from build123d import *

# Parameters (mm, degrees)
SKETCH1_R                = 2.54
BOSS_EXTRUDE1_DEPTH      = 5.08
BOSS_EXTRUDE1_DEPTH_BACK = 5.08
CUT_EXTRUDE1_DEPTH       = 8.981097998
CUT_EXTRUDE1_DEPTH_BACK  = 4.81


with BuildPart() as part:
    # Sketch1 → Boss-Extrude1 (new body, two sides)
    with BuildSketch(Plane(origin=(0, 0, 0), x_dir=(1, 0, 0), z_dir=(0, 1, 0))) as boss_extrude1_sk:
        with BuildLine():
            Line((-2.006502941, 3.238834041), (-11.917388437, -2.901097998))
            Line((-11.917388437, -2.901097998), (-16.997388437, -2.901097998))
            Line((-16.997388437, -2.901097998), (-16.997388437, -7.981097998))
            Line((-16.997388437, -7.981097998), (-11.917388437, -7.981097998))
            Line((-11.917388437, -7.981097998), (0, -3.81))
            Line((0, -3.81), (11.917388437, -7.981097998))
            Line((11.917388437, -7.981097998), (16.997388437, -7.981097998))
            Line((16.997388437, -7.981097998), (16.997388437, -2.901097998))
            Line((16.997388437, -2.901097998), (11.917388437, -2.901097998))
            Line((11.917388437, -2.901097998), (2.006502941, 3.238834041))
            ThreePointArc((2.006502941, 3.238834041), (0, 3.81), (-2.006502941, 3.238834041))
        make_face()
        Circle(SKETCH1_R, mode=Mode.SUBTRACT)
    extrude(amount=BOSS_EXTRUDE1_DEPTH)
    extrude(boss_extrude1_sk.sketch, amount=-BOSS_EXTRUDE1_DEPTH_BACK)

    # Sketch2 → Cut-Extrude1 (cut, two sides)
    with BuildSketch(Plane.XY) as cut_extrude1_sk:
        Polygon((-11.917388437, -6.525255909), (-11.917388437, -2.478330742), (-9.439057695, 0), (9.439057695, 0), (11.917388437, -2.478330742), (11.917388437, -6.525255909), align=None)
        Polygon((-18.093487835, 0), (-11.917388437, 0), (-7.769454267, 4.147934171), (7.769454267, 4.147934171), (11.917388437, 0), (18.118549734, 0), (18.118549734, 7.57171578), (-18.093487835, 7.57171578), align=None)
    extrude(amount=CUT_EXTRUDE1_DEPTH, mode=Mode.SUBTRACT)
    extrude(cut_extrude1_sk.sketch, amount=-CUT_EXTRUDE1_DEPTH_BACK, mode=Mode.SUBTRACT)

    # Sketch3 → Cut-Revolve1 (revolve, cut)
    with BuildSketch(Plane.XY.offset(5.441097998)):
        with BuildLine():
            Line((-12.967633979, -0.885782562), (-12.851197898, -0.885782562))
            Line((-12.851197898, -0.885782562), (-12.851197898, 1.801061794))
            Line((-12.851197898, 1.801061794), (-18.158310447, 1.801061794))
            Line((-18.158310447, 1.801061794), (-18.158310447, -2.54))
            Line((-18.158310447, -2.54), (-16.997388437, -2.54))
            ThreePointArc((-16.997388437, -2.54), (-15.537067777, -0.361964398), (-12.967633979, -0.885782562))
        make_face()
        with BuildLine():
            Line((12.851197898, -0.885782562), (12.851197898, 1.801061794))
            Line((12.851197898, 1.801061794), (18.158310447, 1.801061794))
            Line((18.158310447, 1.801061794), (18.158310447, -2.54))
            Line((18.158310447, -2.54), (16.997388437, -2.54))
            ThreePointArc((16.997388437, -2.54), (15.537067777, -0.361964398), (12.967633979, -0.885782562))
            Line((12.967633979, -0.885782562), (12.851197898, -0.885782562))
        make_face()
    revolve(axis=Axis((-16.997388437, -2.54, 5.441097998), (1, 0, 0)), mode=Mode.SUBTRACT)


solid = part.part
Verification items for the finished model (mm, model axes). A direction names the side the tool comes from. Coordinates: 2 decimals unless noted, no trailing zeros. Order: outer loops, then holes, each group sorted by start corner. A loop starts at its lowest first (then second) coordinate and runs counter-clockwise, first axis right, second up. Notation, with made-up numbers: M 14.25,-27 L 24.25,-27 A5 cw 24.25,-23 Z; hole C -9.5,69 d10. An arc over 180 degrees is marked long. One line per item, written item: value. Start each with the question number.
Item 1: Sectioned sample at D-D on x = -13.5. Record the cut outline in (y, z).
Item 2: Depth check by flat-ended pin: P1, Ø6, axis at x = -3, z = 2.5, coming from the -Y side; P2, Ø3, axis at y = 0.5, z = 6.5, coming from the +X side; P3, Ø0.5, axis at x = -12.5, z = 5.5, coming from the +Y side. Enter the tip coordinate at first touch or a pass-through.
Item 3: Sectioned sample at C-C on z = 2. Record the cut outline in (x, y).
Item 4: Access from +Z, -Z, +X, -X, +Y, -Y to the whole of each face (thin tool, end or side, straight path). Record for faces 4 (the flat face through (12.851, -0.8, 6)), 5 (the flat face through (0, 0, 3)), 6 (the flat face through (-12.4, -2.5, 2.901)).
Item 5: Sectioned sample at A-A on z = 5.75. Record the cut outline in (x, y), then the cut area to 3 significant figures.
Item 6: Sectioned sample at B-B on y = 1.25. Record the cut outline in (x, z), then the cut area to 3 significant figures.
Item 7: Thickness scan on probe 1 along Z at (x, y) = (0, 2.9); probe 2 along X at (y, z) = (2.25, -1.5); probe 3 along Y at (x, z) = (-7, 5). Record the ranges inside material, lowest first.
Item 8: Mould release check, pull along X, two halves, no side actions. Record for faces 1 (the cylindrical face through (0.03, 2.1, -3.81)), 2 (the flat face through (-10.7, -1.26, 4.63)), 3 (the flat face through (12.4, -5.08, 5.4)): pulls with the +X half, pulls with the -X half, needs draft (parallel to the pull), parting line crosses it, or undercut.
Calculated:
1. outline: C -2.54,5.44 d4.12
2. P1: y = 0
2. P2: x = 16.25
2. P3: y = 0
3. outline: M -10.46,-1.02 L -9.44,0 L -1.57,0 L -1.57,4.15 L -7.77,4.15 L -10.46,1.45 Z; M 1.57,0 L 9.44,0 L 10.46,-1.02 L 10.46,1.45 L 7.77,4.15 L 1.57,4.15 Z
4. face 4: none
4. face 5: +Z, -Z, -Y
4. face 6: -Z, -X, +Y, -Y
5. outline: M -12.97,-4.17 L -12.85,-4.17 L -12.85,-5.08 L -11.92,-5.08 L -11.92,-2.48 L -9.44,0 L -5.54,0 L -5.54,4.15 L -7.77,4.15 L -11.92,0 L -12.85,0 L -12.85,-0.91 L -12.97,-0.91 A2.33 ccw long Z; M 5.54,0 L 9.44,0 L 11.92,-2.48 L 11.92,-5.08 L 12.85,-5.08 L 12.85,-4.17 L 12.97,-4.17 A2.33 ccw long 12.97,-0.91 L 12.85,-0.91 L 12.85,0 L 11.92,0 L 7.77,4.15 L 5.54,4.15 Z
5. area: 83.3 mm^2
6. outline: M -10.67,2.13 L -2.01,-3.24 A3.81 ccw 2.01,-3.24 L 10.67,2.13 L 10.67,7.54 L 0,3.81 L -10.67,7.54 Z; hole C 0,0 d5.08
6. area: 125 mm^2
7. probe 1: -3.81 to -2.54, 2.54 to 3.81
7. probe 2: -4.81 to -2.05, 2.05 to 4.81
7. probe 3: 0 to 4.15
8. face 1: parting line crosses it
8. face 2: undercut
8. face 3: needs draft
